Input: part model. Units: mm. Frame: model coordinates. Face numbers are marked on the shaded views. A direction names the side the tool comes from. Coordinates: 2 decimals unless noted, no trailing zeros. Write each loop counter-clockwise with the first axis right and the second up, starting at its lowest first coordinate (ties: lowest second). Pieces come first, ordered by that corner, then holes. Notation, with made-up numbers: (17, -40) - (41, -40) arc R20 cw to (41, -11) - close; hole circle Ø3 at (82.25, -3.5). An arc over 180 degrees is marked (long way). One line per question, with ' | ' between items. Start each with the question number.
1) Section query A-A on z = 22.75. Return loops of the section in (x, y) (3 decimals), and give its area (3 significant figures).
2) Section query B-B on x = -15.5. Return loops of the section in (y, z), and give its area (3 significant figures).
3) Line query: line 1 (X direction, y = 14.5, z = 12.5); line 2 (X direction, y = 1.25, z = 10.25); line 3 (Y direction, x = -17, z = 27.25). Output: solid intervals per line, ascending.
4) Reachability of the marked faces 1, 2, 3, 4 and 5 from +Z, -Z, +X, -X, +Y, -Y: full face, straight path, thin tool, end or side. Return the list, or none.
5) First-contact query: P1, Ø5.5, axis at y = 10.5, z = 19.5, coming from the +X side; P2, Ø5, axis at y = 15.5, z = 13, coming from the -X side; P3, Ø1.6, axis at x = 8, z = 12.5, coming from the -Y side. Flat tips, straight axial feed; report the tip coordinate or a pass-through.
6) Draft query along Y for the marked faces 6, 7, 8 and 9. Return one class per face: released by +Y, released by -Y, zero draft, split by the parting line, or undercut.
7) Section query D-D on x = -29.5. Return loops of the section in (y, z).
8) Section query C-C on y = 1.5. Return loops of the section in (x, z).
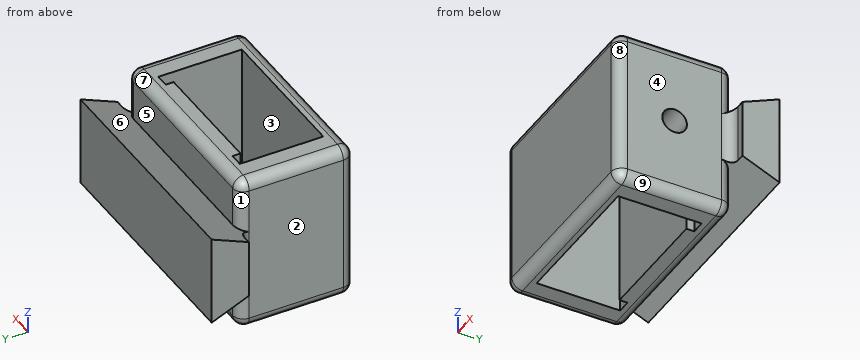
Autodesk Inventor part; units mm, degrees
ref_plane "YZ Plane" through (0, 0, 0) normal (1, 0, 0) x (0, 1, 0)
ref_plane "XZ Plane" through (0, 0, 0) normal (0, 1, 0) x (-1, 0, 0)
ref_plane "XY Plane" through (0, 0, 0) normal (0, 0, 1) x (1, 0, 0)
sketch "Skizze1" plane through (0, 0, 0) normal (0, 0, 1) x (1, 0, 0)
  line L0 (0, 0) -> (-27.75, 0)
  line L1 (-27.75, 0) -> (-27.75, 15.75)
  line L2 (-27.75, 15.75) -> (-25.25, 15.75)
  line L3 (-25.25, 15.75) -> (-25.25, 14.25)
  line L4 (-25.25, 14.25) -> (-2.5, 14.25)
  line L5 (-2.5, 14.25) -> (-2.5, 15.75)
  line L6 (-2.5, 15.75) -> (0, 15.75)
  line L7 (0, 15.75) -> (0, 0)
  line L8 (-32.75, -3) -> (5, -3)
  line L9 (5, -3) -> (5, 18.75)
  line L10 (5, 18.75) -> (-32.75, 18.75)
  line L11 (-32.75, 18.75) -> (-32.75, -3)
  line L12 (-27.75, 7.3651) -> (-32.75, 7.3651)
  line L13 (0, 6.5814) -> (5, 6.5814)
  dimension "d0" = 27.75
  dimension "d1" = 2.5
  dimension "d2" = 1.5
  dimension "d3" = 2.5
  dimension "d4" = 37.75
  dimension "d5" = 3
  dimension "d6" = 3
  dimension "d7" = 15.75
extrude "Extrusion1" add sketch "Skizze1" along normal blind 30 contours L7 L13 L9 L8 L11 L12 L1 L0 | L7 L6 L5 L4 L3 L2 L1 L12 L11 L10 L9 L13
sketch "Skizze2" plane through (-32.75, 18.75, 0) normal (0, 1, 0) x (1, 0, 0)
  line L0 (-3.475, -6.5) -> (41.225, -6.5)
  line L1 (41.225, -6.5) -> (41.225, -23.5)
  line L2 (41.225, -23.5) -> (-3.475, -23.5)
  line L3 (-3.475, -23.5) -> (-3.475, -6.5)
  line L4 (37.75, -30) -> (0, -30)
  line L5 (0, -30) -> (37.75, -30)
  line L6 (0, 0) -> (37.75, 0)
  point P0 (32.75, 0)
  dimension "d10" = 17
  dimension "d14" = 44.7
extrude "Extrusion2" add sketch "Skizze2" along normal blind 7
sketch "Skizze3" plane through (8.475, 18.75, 23.5) normal (1, 0, 0) x (0, 0, -1)
  line L0 (17, 0) -> (0, 0)
  line L1 (0, 0) -> (3, 0)
  line L2 (0, 0) -> (-6.5, 0)
  line L3 (0, 0) -> (0, 7)
  line L4 (0, 0) -> (0, 7)
  line L5 (0, 7) -> (3, 0)
  line L6 (17, 0) -> (14, 0)
  line L7 (14, 0) -> (17, 7)
  line L8 (17, 0) -> (17, 7)
  line L9 (17, 7) -> (17, 0)
  point P0 (23.5, -18.75)
  dimension "d17" = 3
  dimension "d18" = 3
extrude "Extrusion3" cut sketch "Skizze3" against normal through all
sketch "Skizze4" plane through (5, -3, 0) normal (1, 0, 0) x (0, 0, -1)
  circle A0 centre (-15, 10.875) radius 2.325
  line L0 (-15, 10.875) -> (-30, 10.875)
  line L1 (-30, 0) -> (-30, 21.75)
  line L2 (-15, 10.875) -> (-15, 21.75)
  line L3 (-9.5, 21.75) -> (-20.5, 21.75)
  point P0 (0, 3)
  dimension "d21" = 4.65
  dimension "d22" = 90
  dimension "d23" = 90
extrude "Extrusion4" cut sketch "Skizze4" against normal blind 7
fillet "Rundung1" radius 2 6 edges at (-32.75, -3, 15) (5, -3, 15) (5, 18.75, 25.25) (5, 18.75, 4.75) (-32.75, 18.75, 4.75) (-32.75, 18.75, 25.25)
fillet "Rundung2" radius 2 2 edges at (5, 18.75, 15) (-32.75, 18.75, 15)
fillet "Rundung3" radius 2 16 edges at (-32.1642, -2.4142, 30) (-13.875, -3, 30) (4.4142, -2.4142, 30) (5, 7.875, 30) (4.4142, 18.1642, 30) (-13.875, 18.75, 30) (-32.1642, 18.1642, 30) (-32.75, 7.875, 30) (-32.1642, -2.4142, 0) (-13.875, -3, 0) (4.4142, -2.4142, 0) (5, 7.875, 0) (4.4142, 18.1642, 0) (-13.875, 18.75, 0) (-32.1642, 18.1642, 0) (-32.75, 7.875, 0)
properties part number "Schienenläufer_mit_keil_27.5_15.11"
Answer key:
1) outline: (-36.225, 24) - (8.475, 24) - (8.475, 25.75) - (-36.225, 25.75) - close; (-32.75, -1) arc R2 ccw to (-30.75, -3) - (3, -3) arc R2 ccw to (5, -1) - (5, 16.75) arc R2 ccw to (3, 18.75) - (-30.75, 18.75) arc R2 ccw to (-32.75, 16.75) - close; hole (-27.75, 0) - (0, 0) - (0, 15.75) - (-2.5, 15.75) - (-2.5, 14.25) - (-25.25, 14.25) - (-25.25, 15.75) - (-27.75, 15.75) - close | area: 493 mm²
2) outline: (-3, 2) arc R2 ccw to (-1, 0) - (0, 0) - (0, 30) - (-1, 30) arc R2 ccw to (-3, 28) - close; (14.25, 0) - (16.75, 0) arc R2 ccw to (18.75, 2) - (18.75, 9.5) - (25.75, 6.5) - (25.75, 23.5) - (18.75, 20.5) - (18.75, 28) arc R2 ccw to (16.75, 30) - (14.25, 30) - close | area: 320 mm²
3) line 1: -32.75 to -27.75, -25.25 to -2.5, 0 to 5 | line 2: -32.75 to -27.75, 0 to 5 | line 3: -3 to 0, 14.25 to 18.75
4) face 1: +Z, -X | face 2: +Z, -Z, -X, -Y | face 3: +Z, -Z | face 4: +Z, -Z, +X, -Y | face 5: +Z, +X, -X
5) P1: x = 5 | P2: x = -33.19 | P3: y = 18.75
6) face 6: undercut | face 7: released by +Y | face 8: released by -Y | face 9: zero draft
7) outline: (-3, 2) arc R2 ccw to (-1, 0) - (16.75, 0) arc R2 ccw to (18.75, 2) - (18.75, 9.5) - (25.75, 6.5) - (25.75, 23.5) - (18.75, 20.5) - (18.75, 28) arc R2 ccw to (16.75, 30) - (-1, 30) arc R2 ccw to (-3, 28) - close
8) outline: (-32.75, 2) arc R2 ccw to (-30.75, 0) - (-27.75, 0) - (-27.75, 30) - (-30.75, 30) arc R2 ccw to (-32.75, 28) - close; (0, 0) - (3, 0) arc R2 ccw to (5, 2) - (5, 28) arc R2 ccw to (3, 30) - (0, 30) - close
